from build123d import *

# Parameters (mm, degrees)
F1_DEPTH = 20
F2_R     = 3
F3_SIZE2 = 3
F3_SIZE  = 0.5


with BuildPart() as f1:
    # F0 (on Top) → F1 (new body)
    with BuildSketch(Plane.XY):
        with BuildLine():
            Line((17.875, 14.5), (-18.125, 14.5))
            Line((-18.125, 14.5), (-18.125, 6))
            ThreePointArc((-18.125, 6), (-24.125, 0), (-18.125, -6))
            Line((-18.125, -6), (-18.125, -14.5))
            Line((-18.125, -14.5), (17.875, -14.5))
            Line((17.875, -14.5), (17.875, -11.5))
            Line((17.875, -11.5), (26.875, -11.5))
            Line((26.875, -11.5), (26.875, -6.244789))
            ThreePointArc((26.875, -6.244789), (32.869789, -0.25), (26.875, 5.744789))
            Line((26.875, 5.744789), (26.875, 11.25))
            Line((26.875, 11.25), (17.875, 11.25))
            Line((17.875, 11.25), (17.875, 14.5))
        make_face()
        with BuildLine():
            Line((-15.375, 3), (-15.375, 11.75))
            Line((-15.375, 11.75), (15.125, 11.75))
            Line((15.125, 11.75), (15.125, 8.5))
            Line((15.125, 8.5), (24.125, 8.5))
            Line((24.125, 8.5), (24.125, 2.75))
            Line((24.125, 2.75), (26.875, 2.75))
            ThreePointArc((26.875, 2.75), (29.875, -0.25), (26.875, -3.25))
            Line((26.875, -3.25), (24.125, -3.25))
            Line((24.125, -3.25), (24.125, -8.75))
            Line((24.125, -8.75), (15.125, -8.75))
            Line((15.125, -8.75), (15.125, -11.75))
            Line((15.125, -11.75), (-15.375, -11.75))
            Line((-15.375, -11.75), (-15.375, -3))
            Line((-15.375, -3), (-18.125, -3))
            ThreePointArc((-18.125, -3), (-21.125, 0), (-18.125, 3))
            Line((-18.125, 3), (-15.375, 3))
        make_face(mode=Mode.SUBTRACT)
    extrude(amount=F1_DEPTH)

    # F2
    f2_edges = [f1.edges().sort_by_distance(p)[0] for p in [
        (26.875, -6.244789, 10),
        (26.875, 5.744789, 10),
        (-18.125, 6, 10),
        (-18.125, -6, 10),
    ]]
    fillet(f2_edges, radius=F2_R)

    # F3
    f3_edges = [f1.edges().sort_by_distance(p)[0] for p in [
        (-15.375, 7.375, 20),
        (-0.125, 11.75, 20),
        (-15.375, -7.375, 20),
        (-0.125, -11.75, 20),
        (15.125, -10.25, 20),
        (15.125, 10.125, 20),
        (19.625, 8.5, 20),
        (24.125, 5.625, 20),
        (24.125, -6, 20),
        (19.625, -8.75, 20),
    ]]
    chamfer(f3_edges, length=F3_SIZE, length2=F3_SIZE2)


solid = f1.part
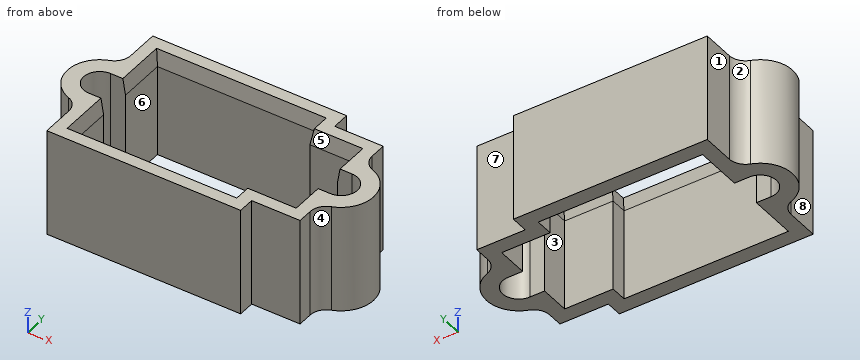
Design review of the part built by this model. Coordinates are the model's own, in mm. Face numbers are marked on the shaded views. A direction names the side the tool comes from. Coordinates: 2 decimals unless noted, no trailing zeros. Loops run counter-clockwise (first coordinate to the right, second up) from the corner with the lowest first, then second, coordinate; pieces in that order, holes last. Notation, with made-up numbers: (66, 23) - (81, 23) arc R20 cw to (81, 40) - close; hole circle Ø9 at (81.5, 66). An arc over 180 degrees is marked (long way). Use CSV: the item, a comma, the result in double quotes. Start each with the question number.
1. Mouldability with a two-part tool opening along Y and no side actions: class the marked faces 1, 2, 3 and 4 as released by +Y, released by -Y, zero draft, split by the parting line, or undercut.
2. Clearance check with flat-ended pins moving along their axes: pin 1 (3 mm diameter, centred on y = -11, z = 14.5, fed in from -X) (3 decimals); pin 2 (3 mm diameter, centred on x = 26, z = 13, fed in from -Y); pin 3 (0.9 mm diameter, centred on y = -13.5, z = 8.5, fed in from +X) (3 decimals). State where each tip first meets the part, or that it passes through.
3. Add section B-B on x = 7. Give the boundary of the cut face in (y, z).
4. To check wall thickness, follow probe 1 along Y at (x, z) = (16.5, 2.5); probe 2 along Y at (x, z) = (-4, 13); probe 3 along X at (y, z) = (11, 2.5) (3 decimals). State the ranges of each line that lie inside material, in increasing order.
5. For the marked faces 5, 6, 7 and 8, list the 3-axis set-ups (+Z, -Z, +X, -X, +Y, -Y) from which the entire face can be reached by the end or side of a thin tool; tool diameter is ignored.
6. Add section A-A on y = 10. Give the boundary of the cut face in (x, z) (3 decimals), plus the area to 4 significant figures.
7. Add section D-D on y = 1.75. Give the boundary of the cut face in (x, z).
Resolved:
1,face 1,"zero draft"
1,face 2,"released by +Y"
1,face 3,"undercut"
1,face 4,"released by -Y"
2,pin 1,"x = -18.125"
2,pin 2,"y = -11.5"
2,pin 3,"x = 17.875"
3,outline,"(-14.5, 0) - (-11.75, 0) - (-11.75, 17) - (-12.25, 20) - (-14.5, 20) - close; (11.75, 0) - (14.5, 0) - (14.5, 20) - (12.25, 20) - (11.75, 17) - close"
4,probe 1,"-14.5 to -8.75, 8.5 to 14.5"
4,probe 2,"-14.5 to -11.75, 11.75 to 14.5"
4,probe 3,"-18.125 to -15.375, 15.125 to 26.875"
5,face 5,"+Z"
5,face 6,"+Z, -Z"
5,face 7,"+Z, -Z, +X, +Y"
5,face 8,"+Z, -Z, -X, -Y"
6,outline,"(-18.125, 0) - (-15.375, 0) - (-15.375, 17) - (-15.875, 20) - (-18.125, 20) - close; (15.125, 0) - (26.875, 0) - (26.875, 20) - (15.625, 20) - (15.125, 17) - close"
6,area,"288.5 mm2"
7,outline,"(-23.86, 0) - (-20.56, 0) - (-20.56, 20) - (-23.86, 20) - close; (29.11, 0) - (32.53, 0) - (32.53, 20) - (29.11, 20) - close"
